Job drawing, mm, ordinate dimensions from the low corner. One solid piece. A direction names the side the tool comes from. Round coordinates to 2 decimals unless told otherwise and drop trailing zeros. Loops run counter-clockwise (first coordinate to the right, second up) from the corner with the lowest first, then second, coordinate; pieces in that order, holes last.
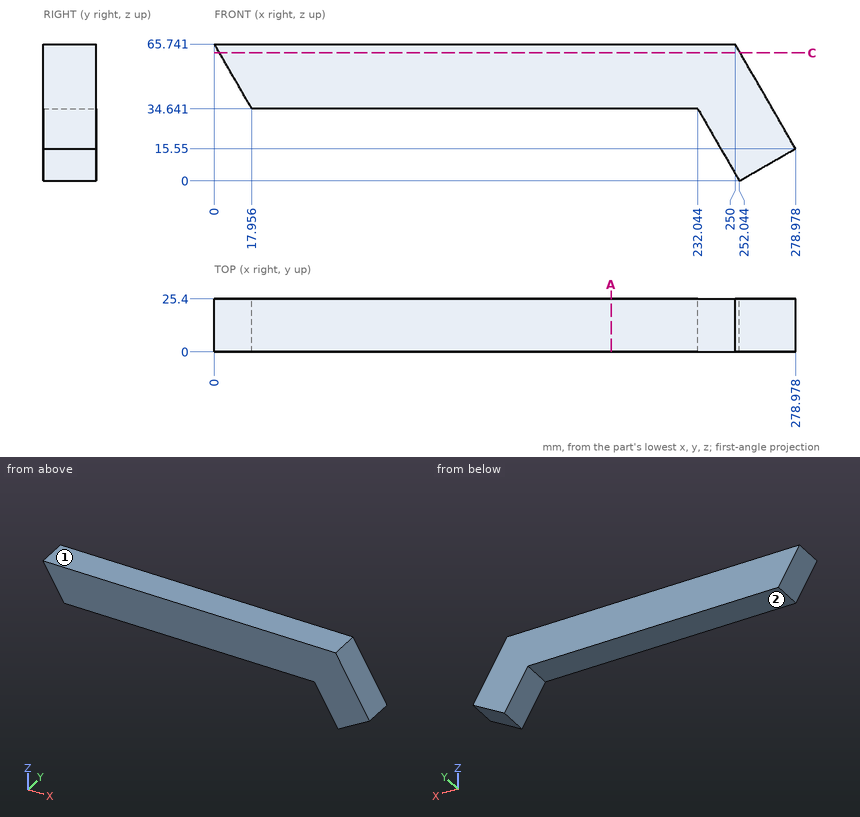
1) Slice it at C-C, the plane z = 61.5. Give the cut face in (x, y).
Values:
outline: (2.45, 0) - (252.45, 0) - (252.45, 25.4) - (2.45, 25.4) - close
2) Tool access for the marked faces 1 and 2: list every direction of +Z, -Z, +X, -X, +Y, -Y with a clear straight run to the whole face (end or side of a thin tool).
Values:
face 1: +Z, +X, -X, +Y, -Y
face 2: -Z, -X, +Y, -Y
3) Wall check: line 1 along Z through (x, y) = (170.5, 18.5); line 2 along X through (y, z) = (11.5, 36); line 3 along X through (y, z) = (5.25, 24). Give the ranges that are in metal, low to high.
Values:
line 1: z = 34.64 to 65.74
line 2: x = 17.17 to 267.17
line 3: x = 238.19 to 274.1
4) Slice it at A-A, the plane x = 190.5. Give the cut face in (y, z).
Values:
outline: (0, 34.64) - (25.4, 34.64) - (25.4, 65.74) - (0, 65.74) - close
5) Drop flat-ended pins along their axis: pin 1 Ø3 at (y, z) = (12.5, 53.5) entering from -X; pin 2 Ø1.5 at (y, z) = (5, 19.5) entering from +X; pin 3 Ø2 at (y, z) = (12, 54.5) entering from -X. Give the stop position or say it passes through.
Values:
pin 1: stops at x = 6.2
pin 2: stops at x = 277.13
pin 3: stops at x = 5.91
